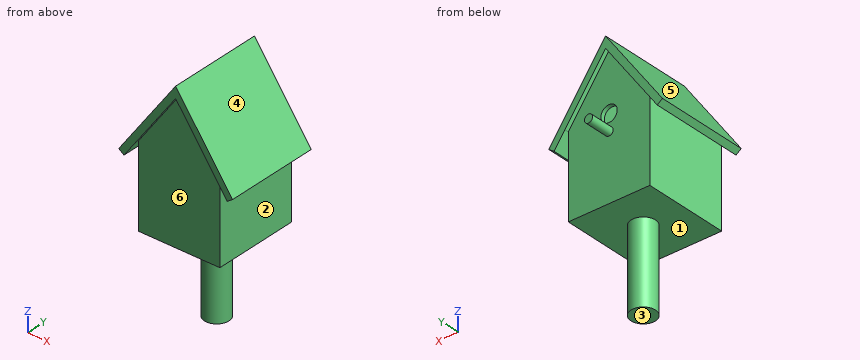
```python
from build123d import *

# Parameters (mm, degrees)
F0_R     = 2.5
F0_R_2   = 5
F1_DEPTH = 2.5
F2_DEPTH = 50
F4_DEPTH = 2.5
F5_DEPTH = 55
F6_DEPTH = 2.5
F7_DEPTH = 15
F8_R     = 7.5
F9_DEPTH = 50


with BuildPart() as f1:
    # F0 (on Front) → F1 (new body)
    with BuildSketch(Plane.XZ):
        Polygon((22.5, 25), (22.5, 28.5), (0, 60), (-22.5, 28.5), (-22.5, 25), (-22.5, -22.5), (22.5, -22.5), align=None)
        with Locations((0, 15)):
            Circle(F0_R, mode=Mode.SUBTRACT)
        with Locations((0, 25)):
            Circle(F0_R_2, mode=Mode.SUBTRACT)
        with Locations((0, 15)):
            Circle(F0_R)
    extrude(amount=F1_DEPTH)

    # F0 (on Front) → F2 (join)
    with BuildSketch(Plane.XZ):
        Polygon((-25, -25), (25, -25), (25, 25), (22.5, 28.5), (22.5, 25), (22.5, -22.5), (-22.5, -22.5), (-22.5, 25), (-22.5, 28.5), (-25, 25), align=None)
    extrude(amount=F2_DEPTH)

    # F3 (on face) → F4 (join)
    with BuildSketch(Plane.XZ.offset(50)):
        Polygon((22.5, 28.5), (22.5, 25), (22.5, -22.5), (-22.5, -22.5), (-22.5, 25), (-22.5, 28.5), (-25, 25), (-25, -25), (25, -25), (25, 25), align=None)
        Polygon((22.5, -22.5), (22.5, 25), (22.5, 28.5), (0, 60), (-22.5, 28.5), (-22.5, 25), (-22.5, -22.5), align=None)
    extrude(amount=F4_DEPTH)

    # F0 (on Front) → F5 (join)
    with BuildSketch(Plane.XZ):
        Polygon((22.5, 28.5), (25, 25), (31.619358, 15.732899), (34.874292, 18.057852), (0, 66.88186), (-34.874292, 18.057852), (-31.619358, 15.732899), (-25, 25), (-22.5, 28.5), (0, 60), align=None)
    extrude(amount=F5_DEPTH)

    # F0 (on Front) → F6 (join)
    with BuildSketch(Plane.XZ):
        Polygon((22.5, 28.5), (25, 25), (31.619358, 15.732899), (34.874292, 18.057852), (0, 66.88186), (-34.874292, 18.057852), (-31.619358, 15.732899), (-25, 25), (-22.5, 28.5), (0, 60), align=None)
    extrude(amount=-F6_DEPTH)

    # F0 (on Front) → F7 (join)
    with BuildSketch(Plane.XZ):
        with Locations((0, 15)):
            Circle(F0_R)
    extrude(amount=-F7_DEPTH)

    # F8 (on face) → F9 (join)
    with BuildSketch(Plane(origin=(0, 0, -25), x_dir=(1, 0, 0), z_dir=(0, 0, -1))):
        with Locations((0, 25)):
            Circle(F8_R)
    extrude(amount=F9_DEPTH)


solid = f1.part
```
Could you check a few things on this model? Use its own coordinates, in mm. Face numbers are marked on the shaded views. A direction names the side the tool comes from. Coordinates: 2 decimals unless noted, no trailing zeros. Write each loop counter-clockwise with the first axis right and the second up, starting at its lowest first coordinate (ties: lowest second). Pieces come first, ordered by that corner, then holes. Notation, with made-up numbers: (-23.5, 40.25) -> (-6.5, 40.25) arc R28 cw to (-6.5, 67.25) -> close; hole circle Ø3 at (-12, -20). An arc over 180 degrees is marked (long way). Write item = value, one per line. Start each with the question number.
(1) Which directions (+Z, -Z, +X, -X, +Y, -Y) give clear straight access to the entire face, cutting with the end or side of a thin tool? Please do the marked faces 1, 2 and 3.
(2) I want a section at B-B (y = -36). Please give me the cut outline in (x, z), plus the area to 3 significant figures.
(3) I need wall thicknesses on line 1 (Y direction, x = -18.5, z = -16); line 2 (X direction, y = -8, z = -4); line 3 (Z direction, x = 0, y = -1.6). Which ranges of each line are inside material? Lowest first, please. Write a range as [from, to].
(4) I want a section at D-D (z = -51.5). Please give me the cut outline in (x, y).
(5) I want a section at A-A (z = 2.5). Please give me the cut outline in (x, y), plus the area to 4 significant figures.
(6) Will these pins go through, and if not, where does the flat tip stop? pin 1 (12 mm diameter, centred on y = -40.5, z = 5.5, fed in from -X); pin 2 (11.5 mm diameter, centred on x = 0, z = 25, fed in from -Y); pin 3 (8 mm diameter, centred on x = 2, z = -37.5, fed in from -Y).
(7) I want a section at C-C (x = 14). Please give me the cut outline in (y, z).
(8) We'd pull the mould along X, two halves only. Please class the marked faces 4, 5 and 6: released by +X, released by -X, zero draft, split by the parting line, or undercut.
Result set:
q1.face_1 = -Z
q1.face_2 = -Z, +Y, -Y
q1.face_3 = -Z, +X, -X, +Y, -Y
q2.outline = (-34.87, 18.06) -> (-31.62, 15.73) -> (-25, 25) -> (-25, -25) -> (25, -25) -> (25, 25) -> (31.62, 15.73) -> (34.87, 18.06) -> (0, 66.88) -> close; hole (-22.5, -22.5) -> (22.5, -22.5) -> (22.5, 28.5) -> (0, 60) -> (-22.5, 28.5) -> close
q2.area = 829 mm2
q3.line_1 = [-52.5, -50], [-2.5, 0]
q3.line_2 = [-25, -22.5], [22.5, 25]
q3.line_3 = [-25, 20], [30, 66.88]
q4.outline = circle Ø15 at (0, -25)
q5.outline = (-25, -52.5) -> (25, -52.5) -> (25, 0) -> (-25, 0) -> close; hole (-22.5, -50) -> (22.5, -50) -> (22.5, -2.5) -> (-22.5, -2.5) -> close
q5.area = 487.5 mm2
q6.pin_1 = -25
q6.pin_2 = -52.5
q6.pin_3 = -32.5
q7.outline = (-55, 40.4) -> (-52.5, 40.4) -> (-52.5, -25) -> (0, -25) -> (0, 40.4) -> (2.5, 40.4) -> (2.5, 47.28) -> (-55, 47.28) -> close; hole (-50, -22.5) -> (-2.5, -22.5) -> (-2.5, 40.4) -> (-50, 40.4) -> close
q8.face_4 = released by +X
q8.face_5 = released by -X
q8.face_6 = undercut
